```python
from build123d import *

# Parameters (mm, degrees)
SKETCH1_R                   = 4.7625
BOSS_EXTRUDE1_DEPTH         = 76.2
SKETCH2_R                   = 4.7625
BOSS_EXTRUDE2_DEPTH         = 38.1
BOSS_EXTRUDE2_TAPER         = 3
F_1_4_28_TAPPED_HOLE1_D     = 5.4102
F_1_4_28_TAPPED_HOLE1_DEPTH = 7.874
F_1_4_28_TAPPED_HOLE1_TIP   = 1.625388061


with BuildPart() as part:
    # Sketch1 → Boss-Extrude1 (new body)
    with BuildSketch(Plane(origin=(0, 0, 0), x_dir=(1, 0, 0), z_dir=(0, 1, 0))):
        with Locations(Location((0, 0, 0), (0, 0, 90))):
            Circle(SKETCH1_R)
    extrude(amount=BOSS_EXTRUDE1_DEPTH)

    # Sketch2 → Boss-Extrude2 (add)
    with BuildSketch(Plane(origin=(0, 76.2, 0), x_dir=(1, 0, 0), z_dir=(0, 1, 0))):
        with Locations(Location((0, 0, 0), (0, 0, 90))):
            Circle(SKETCH2_R)
    extrude(amount=BOSS_EXTRUDE2_DEPTH, taper=BOSS_EXTRUDE2_TAPER)

    # Sketch3 → Revolve1 (revolve)
    with BuildSketch(Plane(origin=(0, 114.3, 0), x_dir=(1, 0, 0), z_dir=(0, 1, 0))):
        with BuildLine():
            Line((0, 2.765763609), (0, -2.765763609))
            ThreePointArc((0, -2.765763609), (2.765763609, 0), (0, 2.765763609))
        make_face()
    revolve(axis=Axis((0, 114.3, -2.765763609), (0, 0, 1)))

    # 1/4-28 Tapped Hole1
    with Locations(Plane.XZ):
        with Locations((0, 0)):
            Hole(F_1_4_28_TAPPED_HOLE1_D / 2, depth=F_1_4_28_TAPPED_HOLE1_DEPTH)
            with Locations((0, 0, -(F_1_4_28_TAPPED_HOLE1_DEPTH + F_1_4_28_TAPPED_HOLE1_TIP / 2))):  # 118° drill point
                Cone(0, F_1_4_28_TAPPED_HOLE1_D / 2, F_1_4_28_TAPPED_HOLE1_TIP, mode=Mode.SUBTRACT)


solid = part.part
```
Check sheet for the modelled part. Datum: model origin and axes. Units: mm. Coordinates: 2 decimals unless noted, no trailing zeros. Write each loop counter-clockwise with the first axis right and the second up, starting at its lowest first coordinate (ties: lowest second). Pieces come first, ordered by that corner, then holes. Notation, with made-up numbers: (46.5, 82.25) -> (69.5, 82.25) arc R26 cw to (69.5, 118.25) -> close; hole circle Ø3 at (-39.75, 77.25). An arc over 180 degrees is marked (long way). Use a Markdown table: item, result.
1. Scan lines: line 1 along X through (y, z) = (1.5, 0); line 2 along Z through (x, y) = (-0.75, 7); line 3 along Y through (x, z) = (2.5, -0.25). Record each from-to range of solid material in increasing order.
Reported:
| item | result |
|---|---|
| line 1 | x = -4.76 to -2.71, 2.71 to 4.76 |
| line 2 | z = -4.7 to -2.6, 2.6 to 4.7 |
| line 3 | y = 7.99 to 115.46 |
2. Go/stop test with flat-tipped pins: pin 1 Ø2 at (x, y) = (-3.5, 101.5) entering from +Z; pin 2 Ø3 at (x, y) = (0, 81.5) entering from +Z; pin 3 Ø1.5 at (x, y) = (-3.5, 104) entering from -Z. Record where each tip stops, or that it passes through.
Reported:
| item | result |
|---|---|
| pin 1 | stops at z = 2.36 |
| pin 2 | stops at z = 4.56 |
| pin 3 | stops at z = -1.84 |
3. Release check for a two-part mould opening along X. For faces 1 (the cylindrical face through (2.9, 37.57, 3.78)), 2 (the cylindrical face through (-2.58, 3.99, 0.81)), 3 (the flat face through (2.05, 0, -2.05)) record: pulls with the +X half, pulls with the -X half, needs draft (parallel to the pull), parting line crosses it, or undercut.
Reported:
| item | result |
|---|---|
| face 1 | parting line crosses it |
| face 2 | undercut |
| face 3 | needs draft |
4. Sectioned sample at B-B (y = 93). Enter the section's corners in (x, z).
Reported:
| item | result |
|---|---|
| outline | circle Ø7.76 at (0, 0) |
5. Sectioned sample at A-A (y = 31.5). Enter the section's corners in (x, z) (1 decimal), plus the area to 3 significant figures.
Reported:
| item | result |
|---|---|
| outline | circle Ø9.5 at (0, 0) |
| area | 71.3 mm2 |
